```python
from build123d import *

# Parameters (mm, degrees)
F0_W     = 187.8524124622
F0_H     = 99.6085852385
F0_W_2   = 171.8524098396
F0_H_2   = 83.6085826159
F1_DEPTH = 97.8
F3_DEPTH = 187.8534124622
F4_W     = 85.7032239437
F4_H     = 39.1587115705
F5_DEPTH = 99.6095852385


with BuildPart() as f1:
    # F0 (on Top) → F1 (new body)
    with BuildSketch(Plane.XY):
        Rectangle(F0_W, F0_H)
        Rectangle(F0_W_2, F0_H_2, mode=Mode.SUBTRACT)
    extrude(amount=F1_DEPTH)

    # F2 (on face) → F3 (cut, through all)
    with BuildSketch(Plane.YZ.offset(93.9262062311)):
        with BuildLine():
            Line((0, 48.9), (-8.06236551, 56.8159777743))
            ThreePointArc((-8.06236551, 56.8159777743), (-11.2988690469, 48.9), (-8.06236551, 40.9840222257))
            Line((-8.06236551, 40.9840222257), (0, 48.9))
        make_face()
        with BuildLine():
            Line((8.06236551, 40.9840222257), (0, 48.9))
            Line((0, 48.9), (-8.06236551, 40.9840222257))
            ThreePointArc((-8.06236551, 40.9840222257), (0, 37.6011309531), (8.06236551, 40.9840222257))
        make_face()
        with BuildLine():
            Line((8.06236551, 56.8159777743), (0, 48.9))
            Line((0, 48.9), (8.06236551, 40.9840222257))
            ThreePointArc((8.06236551, 40.9840222257), (10.4584906618, 44.6239720748), (11.2988690469, 48.9))
            ThreePointArc((11.2988690469, 48.9), (10.4584906618, 53.1760279252), (8.06236551, 56.8159777743))
        make_face()
        with BuildLine():
            ThreePointArc((8.06236551, 56.8159777743), (0, 60.1988690469), (-8.06236551, 56.8159777743))
            Line((-8.06236551, 56.8159777743), (0, 48.9))
            Line((0, 48.9), (8.06236551, 56.8159777743))
        make_face()
    extrude(amount=-F3_DEPTH, mode=Mode.SUBTRACT)

    # F4 (on face) → F5 (cut, through all)
    with BuildSketch(Plane.XZ.offset(49.8042926192)):
        with Locations((0, 78.2206442147)):
            Rectangle(F4_W, F4_H)
    extrude(amount=-F5_DEPTH, mode=Mode.SUBTRACT)


solid = f1.part
```
The listing builds one solid part. Answer for the finished solid, in the listing's coordinates (mm). A direction names the side the tool comes from. Give positions to 0.01 mm unless a question says otherwise; leave off trailing zeros. Order: outer loops, then holes, each group sorted by start corner. A loop starts at its lowest first (then second) coordinate and runs counter-clockwise, first axis right, second up. Notation, with made-up numbers: (-33.5, 10) - (15.5, 10) arc R25 cw to (15.5, 35) - close; hole circle Ø10 at (53, 65.5). An arc over 180 degrees is marked (long way). Answer in a Markdown table with one row per item. Add a question column.
Q1. Which of the six approach directions +Z, -Z, +X, -X, +Y, -Y give full straight-line access (tool end or side, diameter ignored) to faces 5 (the flat face through (-1, 49.804, 37)), 6 (the flat face through (-42.852, -46, 78)), 7 (the flat face through (85.926, -1, 37))?
Q2. The part is cut by section C-C (x = -73.5). Determine the outline of the cut face in (y, z), then the cut area to 3 significant figures.
Q3. The part is cut by section B-B (y = 29). Determine the outline of the cut face in (x, z), then the cut area to 3 significant figures.
Q4. The part is cut by section A-A (z = 90). Determine the outline of the cut face in (x, y), then the cut area to 3 significant figures.
Q5. Find the intervals of material crossed by line 1 along X through (y, z) = (11, 69); line 2 along Y through (x, z) = (56.5, 59); line 3 along Z through (x, y) = (40, 44), in increasing order. Write a range as [from, to].
Q6. The part is cut by section D-D (z = 31.5). Determine the outline of the cut face in (x, y), then the cut area to 3 significant figures.
Q7. For a pull along Y with two mould halves and no side action, classify faces 1 (the flat face through (42.852, -46, 78)), 2 (the flat face through (-1, -41.804, 37)), 3 (the flat face through (-1, -49.804, 37)), 4 (the flat face through (-85.926, -1, 37)) as released by +Y, released by -Y, zero draft, split by the parting line, or undercut.
Q8. Given P1, Ø2.5, axis at x = 16.5, y = 45.5, coming from the +Z side, flat-ended and moving along its own axis, determine where the tip first touches the part or whether it passes through.
Determined:
| question | item | result |
|---|---|---|
| 1 | face 5 | +Z, -Z, +X, -X, +Y |
| 1 | face 6 | +Z, +Y, -Y |
| 1 | face 7 | +Z, -Z |
| 2 | outline | (-49.8, 0) - (-41.8, 0) - (-41.8, 97.8) - (-49.8, 97.8) - close; (41.8, 0) - (49.8, 0) - (49.8, 97.8) - (41.8, 97.8) - close |
| 2 | area | 1,560 mm² |
| 3 | outline | (-93.93, 0) - (-85.93, 0) - (-85.93, 97.8) - (-93.93, 97.8) - close; (85.93, 0) - (93.93, 0) - (93.93, 97.8) - (85.93, 97.8) - close |
| 3 | area | 1,560 mm² |
| 4 | outline | (-93.93, -49.8) - (-42.85, -49.8) - (-42.85, -41.8) - (-85.93, -41.8) - (-85.93, 41.8) - (-42.85, 41.8) - (-42.85, 49.8) - (-93.93, 49.8) - close; (42.85, -49.8) - (93.93, -49.8) - (93.93, 49.8) - (42.85, 49.8) - (42.85, 41.8) - (85.93, 41.8) - (85.93, -41.8) - (42.85, -41.8) - close |
| 4 | area | 2,970 mm² |
| 5 | line 1 | x = [-93.93, -85.93], [85.93, 93.93] |
| 5 | line 2 | y = [-49.8, -41.8], [41.8, 49.8] |
| 5 | line 3 | z = [0, 58.64] |
| 6 | outline | (-93.93, -49.8) - (93.93, -49.8) - (93.93, 49.8) - (-93.93, 49.8) - close; hole (-85.93, -41.8) - (85.93, -41.8) - (85.93, 41.8) - (-85.93, 41.8) - close |
| 6 | area | 4,340 mm² |
| 7 | face 1 | zero draft |
| 7 | face 2 | undercut |
| 7 | face 3 | released by -Y |
| 7 | face 4 | undercut |
| 8 | P1 | stops at z = 58.64 |
